from build123d import *

# Parameters (mm, degrees)
SKETCH2_W               = 266.7
SKETCH2_H               = 1016
BOSS_EXTRUDE1_DEPTH     = 6.35
CUT_EXTRUDE3_DEPTH      = 1025.733402028
CUT_EXTRUDE3_DEPTH_BACK = 1025.733402028
SKETCH5_W               = 12.7
SKETCH5_H               = 508
MOVE_FACE_SLOT_BY       = 0.762
MOVE_FACE_SLOT_2_BY     = 0.762
MOVE_FACE_SLOT_3_BY     = 0.762
FILLET1_R               = 3.175


with BuildPart() as part:
    # Sketch2 → Boss-Extrude1 (new, symmetric)
    with BuildSketch(Plane.XY):
        with Locations((0, 508)):
            Rectangle(SKETCH2_W, SKETCH2_H)
    extrude(amount=BOSS_EXTRUDE1_DEPTH, both=True)

    # Cavity1: read off the stored shape, not the designer's step
    # Cavity1: loft between two sections, ruled curve by curve
    cavity1_from = [
        Edge.make_three_point_arc((-82.55, 819.9, 6.35), (-69.85, 832.6, 6.35), (-57.15, 819.9, 6.35)),
        Edge.make_three_point_arc((-57.15, 819.9, 6.35), (-69.85, 807.2, 6.35), (-82.55, 819.9, 6.35)),
    ]
    cavity1_to = [
        Edge.make_three_point_arc((-82.55, 819.9, -6.35), (-69.85, 832.6, -6.35), (-57.15, 819.9, -6.35)),
        Edge.make_three_point_arc((-57.15, 819.9, -6.35), (-69.85, 807.2, -6.35), (-82.55, 819.9, -6.35)),
    ]
    cavity1 = Solid(Shell([*[Face.make_surface_from_curves(cavity1_from[k], cavity1_to[k]) for k in range(2)], Face(Wire(cavity1_from)), Face(Wire(cavity1_to))]))
    add(cavity1, mode=Mode.SUBTRACT)

    # Cavity1 2: loft between two sections, ruled curve by curve
    cavity1_2_from = [
        Edge.make_three_point_arc((-69.85, 714.991315977, 23.190482806), (-82.55, 724.54904, 14.827474286), (-69.85, 734.106764023, 6.464465766)),
        Edge.make_three_point_arc((-69.85, 734.106764023, 6.464465766), (-57.15, 724.54904, 14.827474286), (-69.85, 714.991315977, 23.190482806)),
    ]
    cavity1_2_to = [
        Edge.make_three_point_arc((-69.85, 689.13960738, -6.354327019), (-82.55, 698.697331403, -14.717335539), (-69.85, 708.255055426, -23.080344059)),
        Edge.make_three_point_arc((-69.85, 708.255055426, -23.080344059), (-57.15, 698.697331403, -14.717335539), (-69.85, 689.13960738, -6.354327019)),
    ]
    cavity1_2 = Solid(Shell([*[Face.make_surface_from_curves(cavity1_2_from[k], cavity1_2_to[k]) for k in range(2)], Face(Wire(cavity1_2_from)), Face(Wire(cavity1_2_to))]))
    add(cavity1_2, mode=Mode.SUBTRACT)

    # Cavity1 3: loft between two sections, ruled curve by curve
    cavity1_3_from = [
        Edge.make_three_point_arc((-82.55, 469.9, 6.35), (-69.85, 482.6, 6.35), (-57.15, 469.9, 6.35)),
        Edge.make_three_point_arc((-57.15, 469.9, 6.35), (-69.85, 457.2, 6.35), (-82.55, 469.9, 6.35)),
    ]
    cavity1_3_to = [
        Edge.make_three_point_arc((-82.55, 469.9, -6.35), (-69.85, 482.6, -6.35), (-57.15, 469.9, -6.35)),
        Edge.make_three_point_arc((-57.15, 469.9, -6.35), (-69.85, 457.2, -6.35), (-82.55, 469.9, -6.35)),
    ]
    cavity1_3 = Solid(Shell([*[Face.make_surface_from_curves(cavity1_3_from[k], cavity1_3_to[k]) for k in range(2)], Face(Wire(cavity1_3_from)), Face(Wire(cavity1_3_to))]))
    add(cavity1_3, mode=Mode.SUBTRACT)

    # Sketch5 → Cut-Extrude3 (cut, two sides: drawn at the far end of the back side and taken through both)
    with BuildSketch(Plane.XY.offset(-CUT_EXTRUDE3_DEPTH_BACK)):
        with Locations((63.5, 762)):
            Rectangle(SKETCH5_W, SKETCH5_H)
    extrude(amount=CUT_EXTRUDE3_DEPTH + CUT_EXTRUDE3_DEPTH_BACK, mode=Mode.SUBTRACT)

    # Move Face slot: a face moved inward by 0.762
    extrude(part.faces().sort_by_distance((63.5, 508, 0))[0], amount=MOVE_FACE_SLOT_BY, dir=(0, -1, 0), mode=Mode.SUBTRACT)

    # Move Face slot 2: a face moved inward by 0.762
    extrude(part.faces().sort_by_distance((69.85, 762, 0))[0], amount=MOVE_FACE_SLOT_2_BY, dir=(1, 0, 0), mode=Mode.SUBTRACT)

    # Move Face slot 3: a face moved inward by 0.762
    extrude(part.faces().sort_by_distance((57.15, 762, 0))[0], amount=MOVE_FACE_SLOT_3_BY, dir=(-1, 0, 0), mode=Mode.SUBTRACT)

    # Fillet1
    fillet1_edges = [part.edges().sort_by_distance(p)[0] for p in [
        (70.612, 1016, 0),
        (70.612, 507.238, 0),
        (56.388, 507.238, 0),
        (56.388, 1016, 0),
    ]]
    fillet(fillet1_edges, radius=FILLET1_R)

    # Move Face hole: read off the stored shape, not the designer's step
    # Move Face hole: loft between two sections, ruled curve by curve
    move_face_hole_from = [
        Edge.make_three_point_arc((-83.185, 819.9, 6.35), (-69.85, 833.235, 6.35), (-56.515, 819.9, 6.35)),
        Edge.make_three_point_arc((-56.515, 819.9, 6.35), (-69.85, 806.565, 6.35), (-83.185, 819.9, 6.35)),
    ]
    move_face_hole_to = [
        Edge.make_three_point_arc((-83.185, 819.9, -6.35), (-69.85, 833.235, -6.35), (-56.515, 819.9, -6.35)),
        Edge.make_three_point_arc((-56.515, 819.9, -6.35), (-69.85, 806.565, -6.35), (-83.185, 819.9, -6.35)),
    ]
    move_face_hole = Solid(Shell([*[Face.make_surface_from_curves(move_face_hole_from[k], move_face_hole_to[k]) for k in range(2)], Face(Wire(move_face_hole_from)), Face(Wire(move_face_hole_to))]))
    add(move_face_hole, mode=Mode.SUBTRACT)

    # Move Face hole 2: loft between two sections, ruled curve by curve
    move_face_hole_2_from = [
        Edge.make_three_point_arc((-69.85, 714.884319276, 24.032506946), (-83.185, 724.9199295, 15.251348), (-69.85, 734.955539724, 6.470189054)),
        Edge.make_three_point_arc((-69.85, 734.955539724, 6.470189054), (-56.515, 724.9199295, 15.251348), (-69.85, 714.884319276, 24.032506946)),
    ]
    move_face_hole_2_to = [
        Edge.make_three_point_arc((-69.85, 688.295650249, -6.35454337), (-83.185, 698.331260473, -15.135702316), (-69.85, 708.366870697, -23.916861262)),
        Edge.make_three_point_arc((-69.85, 708.366870697, -23.916861262), (-56.515, 698.331260473, -15.135702316), (-69.85, 688.295650249, -6.35454337)),
    ]
    move_face_hole_2 = Solid(Shell([*[Face.make_surface_from_curves(move_face_hole_2_from[k], move_face_hole_2_to[k]) for k in range(2)], Face(Wire(move_face_hole_2_from)), Face(Wire(move_face_hole_2_to))]))
    add(move_face_hole_2, mode=Mode.SUBTRACT)

    # Move Face hole 3: loft between two sections, ruled curve by curve
    move_face_hole_3_from = [
        Edge.make_three_point_arc((-83.185, 469.9, 6.35), (-69.85, 483.235, 6.35), (-56.515, 469.9, 6.35)),
        Edge.make_three_point_arc((-56.515, 469.9, 6.35), (-69.85, 456.565, 6.35), (-83.185, 469.9, 6.35)),
    ]
    move_face_hole_3_to = [
        Edge.make_three_point_arc((-83.185, 469.9, -6.35), (-69.85, 483.235, -6.35), (-56.515, 469.9, -6.35)),
        Edge.make_three_point_arc((-56.515, 469.9, -6.35), (-69.85, 456.565, -6.35), (-83.185, 469.9, -6.35)),
    ]
    move_face_hole_3 = Solid(Shell([*[Face.make_surface_from_curves(move_face_hole_3_from[k], move_face_hole_3_to[k]) for k in range(2)], Face(Wire(move_face_hole_3_from)), Face(Wire(move_face_hole_3_to))]))
    add(move_face_hole_3, mode=Mode.SUBTRACT)


solid = part.part
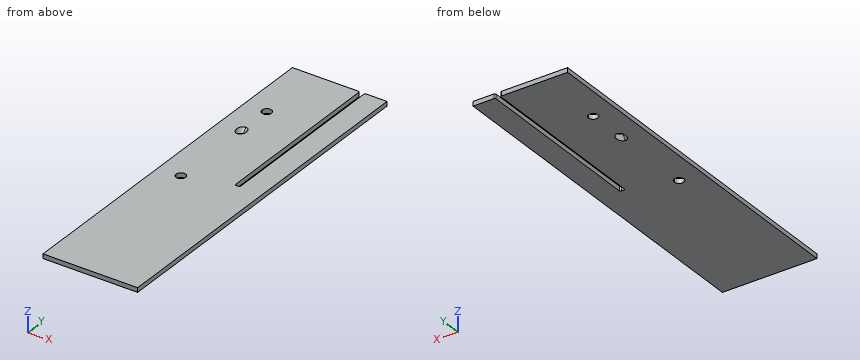
CAD build for the part. Positions are in the model's coordinates, mm. Coordinates: 2 decimals unless noted, no trailing zeros. Loops run counter-clockwise (first coordinate to the right, second up) from the corner with the lowest first, then second, coordinate; pieces in that order, holes last. Notation, with made-up numbers: (89, -30.5) - (103, -30.5) arc R26 cw to (103, 8.5) - close; hole circle Ø7 at (51, 35.5). An arc over 180 degrees is marked (long way). Use one line per item in the form item = value. Start each with the question number.
1) Band-saw the part on B-B (z = -4.25). State how many separate pieces and enclosed holes the cut face has, and give its area (3 significant figures).
2) Flat gauge pin, fed straight in: pin 1 (6.5 mm diameter, centred on x = 62.5, z = -0.5, fed in from +Y). Where does the tip first touch, or does it go through?
3) Drill centre lines: L1, parallel to X at y = 908.5, z = 3.25; L2, parallel to Y at x = -64, z = -1; L3, parallel to Y at x = 57.5, z = 1. Where is each one in solid material? Low to high. Write a range as from..to.
4) Band-saw the part on A-A (y = 949). Give the cut face in (x, z), and give its area (3 significant figures).
Check values:
q1.separate_pieces = 1
q1.enclosed_holes = 3
q1.area = 262,000 mm2
q2.pin_1 = 507.25
q3.L1 = -133.35..56.39, 70.61..133.35
q3.L2 = 0..457.92, 481.88..694.78, 726.62..807.92, 831.88..1016
q3.L3 = 0..508
q4.outline = (-133.35, -6.35) - (56.39, -6.35) - (56.39, 6.35) - (-133.35, 6.35) - close; (70.61, -6.35) - (133.35, -6.35) - (133.35, 6.35) - (70.61, 6.35) - close
q4.area = 3,210 mm2
